```python
from build123d import *

# Parameters (mm, degrees)
SKETCH1_R           = 41.91
SKETCH1_R_2         = 2.4892
SKETCH1_R_3         = 11.938
BOSS_EXTRUDE1_DEPTH = 9.525


with BuildPart() as part:
    # Sketch1 → Boss-Extrude1 (new body)
    with BuildSketch(Plane.XZ):
        Circle(SKETCH1_R)
        with Locations((-20.622229928, -11.90625)):
            Circle(SKETCH1_R_2, mode=Mode.SUBTRACT)
        with Locations((-20.622229928, 11.90625)):
            Circle(SKETCH1_R_2, mode=Mode.SUBTRACT)
        with Locations((0, 23.8125)):
            Circle(SKETCH1_R_2, mode=Mode.SUBTRACT)
        with Locations((20.622229928, 11.90625)):
            Circle(SKETCH1_R_2, mode=Mode.SUBTRACT)
        with Locations((20.622229928, -11.90625)):
            Circle(SKETCH1_R_2, mode=Mode.SUBTRACT)
        Circle(SKETCH1_R_3, mode=Mode.SUBTRACT)
        with Locations((0, -23.8125)):
            Circle(SKETCH1_R_2, mode=Mode.SUBTRACT)
    extrude(amount=-BOSS_EXTRUDE1_DEPTH)


solid = part.part
```
CAD build for the part. Positions are in the model's coordinates, mm. Coordinates: 2 decimals unless noted, no trailing zeros. Write each loop counter-clockwise with the first axis right and the second up, starting at its lowest first coordinate (ties: lowest second). Pieces come first, ordered by that corner, then holes.
(1) Cut at C-C, the plane y = 1. List the corners of the cut face in (x, z), and give its area (3 significant figures).
(2) Cut at A-A, the plane z = 0. List the corners of the cut face in (x, y) (3 decimals).
(3) Flat gauge pins, fed straight in: pin 1 (1 mm diameter, centred on x = -2.5, y = 3.5, fed in from -Z); pin 2 (5 mm diameter, centred on x = -28, y = 2.5, fed in from +Z); pin 3 (2 mm diameter, centred on y = 2, z = -17, fed in from -X). Where does each tip first touch, or does it go through?
(4) Cut at B-B, the plane x = 0. List the corners of the cut face in (y, z) (3 decimals).
(5) Drill centre lines: probe 1 along Z at (x, y) = (0, 6.5); probe 2 along X at (y, z) = (5.25, -2); probe 3 along X at (y, z) = (8.5, 13.5). Where is each one in solid material? Low to high.
(6) Cut at D-D, the plane z = 33. List the corners of the cut face in (x, y) (3 decimals).
(7) Two-plate mould, pull along X, no slides. Class faces 1 (the face through (-5.456, 4.696, 41.553)), 2 (the face through (9, 9.525, -9)), 3 (the face through (-0.54, 4.696, -26.243)): +X half, -X half, draft (parallel to the pull), parting line (faces both ways), or undercut.
Geometry says:
1. outline: circle Ø83.82 at (0, 0); hole circle Ø4.98 at (-20.62, -11.91); hole circle Ø4.98 at (-20.62, 11.91); hole circle Ø23.88 at (0, 0); hole circle Ø4.98 at (0, -23.81); hole circle Ø4.98 at (0, 23.81); hole circle Ø4.98 at (20.62, -11.91); hole circle Ø4.98 at (20.62, 11.91)
1. area: 4,950 mm2
2. outline: (-41.91, 0) - (-11.938, 0) - (-11.938, 9.525) - (-41.91, 9.525) - close; (11.938, 0) - (41.91, 0) - (41.91, 9.525) - (11.938, 9.525) - close
3. pin 1: stops at z = -41.86
3. pin 2: stops at z = 33.26
3. pin 3: stops at x = -38.74
4. outline: (0, -41.91) - (9.525, -41.91) - (9.525, -26.302) - (0, -26.302) - close; (0, -21.323) - (9.525, -21.323) - (9.525, -11.938) - (0, -11.938) - close; (0, 11.938) - (9.525, 11.938) - (9.525, 21.323) - (0, 21.323) - close; (0, 26.302) - (9.525, 26.302) - (9.525, 41.91) - (0, 41.91) - close
5. probe 1: z = -41.91 to -26.3, -21.32 to -11.94, 11.94 to 21.32, 26.3 to 41.91
5. probe 2: x = -41.86 to -11.77, 11.77 to 41.86
5. probe 3: x = -39.68 to -22.53, -18.71 to 18.71, 22.53 to 39.68
6. outline: (-25.835, 0) - (25.835, 0) - (25.835, 9.525) - (-25.835, 9.525) - close
7. face 1: parting line
7. face 2: draft
7. face 3: undercut
